from build123d import *

# Parameters (mm, degrees)
SKETCH_4_R          = 3
CUT_EXTRUDE_1_DEPTH = 15


with BuildPart() as part:
    # 草图1 → 旋转1 (revolve)
    with BuildSketch(Plane.XY):
        with BuildLine():
            Line((-5.454356057, 2.5), (-7.599342077, 2.5))
            ThreePointArc((-7.599342077, 2.5), (-6.480740698, -4.69041576), (0, -8))
            Line((0, -8), (0, -6))
            ThreePointArc((0, -6), (-5.049752469, -3.240370349), (-5.454356057, 2.5))
        make_face()
    revolve(axis=Axis((0, 0, 0), (0, -1, 0)))

    # 草图2 → 旋转2 (revolve)
    with BuildSketch(Plane.XY, mode=Mode.PRIVATE) as revolve_2_sk:
        Polygon((-7.5, 0), (-7.5, 1), (-12.26701437, 5), (-30, 5), (-30, 0), align=None)
    revolve(revolve_2_sk.sketch.rotate(Axis((-7.5, 0, 0), (-1, 0, 0)), 180), axis=Axis((-7.5, 0, 0), (-1, 0, 0)))

    # 草图4 → 切除-拉伸1 (cut)
    with BuildSketch(Plane.ZY.offset(30)):
        with Locations(Location((0, 0, 0), (0, 0, 270))):
            Circle(SKETCH_4_R)
    extrude(amount=-CUT_EXTRUDE_1_DEPTH, mode=Mode.SUBTRACT)


solid = part.part
Geometry check sheet. Reference: the model listing, model coordinates, mm. A direction names the side the tool comes from. Round coordinates to 2 decimals unless told otherwise and drop trailing zeros. Order: outer loops, then holes, each group sorted by start corner. A loop starts at its lowest first (then second) coordinate and runs counter-clockwise, first axis right, second up. Notation, with made-up numbers: (82, 78) - (137, 78) arc R13 ccw to (137, 92) - close; hole circle Ø10 at (71.5, -21.75). An arc over 180 degrees is marked (long way). One line per question, with ' | ' between items. Start each with the question number.
(1) Sectioned sample at B-B on z = 0. Record the cut outline in (x, y).
(2) Depth check by flat-ended pin: pin 1 Ø1.8 at (y, z) = (0, -1) entering from -X; pin 2 Ø4 at (y, z) = (1, 3.5) entering from +X; pin 3 Ø4 at (x, z) = (-13, -4) entering from -Y; pin 4 Ø7 at (y, z) = (0, 0) entering from -X. Enter the tip coordinate at first touch or a pass-through.
(3) Sectioned sample at C-C on x = -0.5. Record the cut outline in (y, z), and give its area (3 significant figures).
(4) Release check for a two-part mould opening along Y. For faces 4 (the flat face through (-30, -3.3, 0.1)), 5 (the cylindrical face through (-21, 5, 0)), 6 (the flat face through (-15, 0, 0)) record: released by +Y, released by -Y, zero draft, split by the parting line, or undercut.
(5) Thickness scan on L1, parallel to Z at x = -24.75, y = 0; L2, parallel to X at y = -4.75, z = 1; L3, parallel to X at y = -2, z = -4.5. Record the ranges inside material, lowest first. Write a range as [from, to].
(6) Sectioned sample at D-D on y = -5.5. Record the cut outline in (x, z), and give its area (3 significant figures).
(7) Sectioned sample at A-A on y = 0. Record the cut outline in (x, z).
(8) Access from +Z, -Z, +X, -X, +Y, -Y to the whole of each face (thin tool, end or side, straight path). Record for faces 1 (the cylindrical face through (-22.6, -2.86, 0.9)), 2 (the conical face through (-8.6, -0.9, -1.7)), 3 (the flat face through (5, 2.5, 3)).
Conclusion:
1) outline: (-30, -5) - (-12.27, -5) - (-7.89, -1.33) arc R8 ccw (long way) to (7.6, 2.5) - (5.45, 2.5) arc R6 cw (long way) to (-5.45, 2.5) - (-7.6, 2.5) arc R8 ccw to (-7.89, 1.33) - (-12.27, 5) - (-30, 5) - (-30, 3) - (-15, 3) - (-15, -3) - (-30, -3) - close
2) pin 1: stops at x = -15 | pin 2: stops at x = 7.83 | pin 3: stops at y = -4.58 | pin 4: stops at x = -30
3) outline: (2.5, -7.58) - (2.5, -5.43) arc R5.98 cw (long way) to (2.5, 5.43) - (2.5, 7.58) arc R7.98 ccw (long way) to start | area: 54.2 mm2
4) face 4: zero draft | face 5: split by the parting line | face 6: undercut
5) L1: z = [-5, -3], [3, 5] | L2: x = [-30, -12.09], [-6.36, -3.53], [3.53, 6.36] | L3: x = [-30, -12.18], [-6.3, -3.43], [3.43, 6.3]
6) outline: circle Ø11.62 at (0, 0); hole circle Ø4.8 at (0, 0) | area: 88.0 mm2
7) outline: (-30, -5) - (-12.27, -5) - (-7.89, -1.33) arc R8 ccw (long way) to (-7.89, 1.33) - (-12.27, 5) - (-30, 5) - (-30, 3) - (-15, 3) - (-15, -3) - (-30, -3) - close; hole circle Ø12 at (0, 0)
8) face 1: -X | face 2: none | face 3: +Z, -Z, +X, +Y
